Read the model definition and answer for the solid it produces. Units are mm, in the model's axes. A direction names the side the tool comes from. Coordinates: 2 decimals unless noted, no trailing zeros. Write each loop counter-clockwise with the first axis right and the second up, starting at its lowest first coordinate (ties: lowest second). Pieces come first, ordered by that corner, then holes. Notation, with made-up numbers: (-1.75, 41) -> (55.25, 41) arc R20 ccw to (55.25, 61) -> close; hole circle Ø7 at (2, 67). An arc over 180 degrees is marked (long way). One line per item, written item: value. Start each with the question number.
1. Find section B-B, the plane y = -48. Write down the section's boundary in (x, z), and give its area (3 significant figures).
2. Find section D-D, the plane y = -9. Write down the section's boundary in (x, z).
3. Given P1, Ø5, axis at x = 12.5, z = 7, coming from the +Y side; P2, Ø6.5, axis at y = -29.5, z = 1.5, coming from the +X side; P3, Ø3, axis at y = -11, z = 0, coming from the -X side, each flat-ended and moving along its own axis, determine where each tip first touches the part or whether it passes through.
4. For faces 5 (the cylindrical face through (40.59, -24.45, 4.93)), 6 (the flat face through (0.62, -46.16, 13.51)), 7 (the cylindrical face through (0.47, -24.79, 4.93)), 8 (the flat face through (0.1, -46.7, 12.5)), determine the directions among +Z, -Z, +X, -X, +Y, -Y from which every point of the face is accessible in a straight line to the end or side of a thin tool.
5. Find section A-A, the plane z = 1. State how many separate pieces and enclosed holes the cut face has, and give its area (3 significant figures).
6. Consider line 1 along Y through (x, z) = (38.5, 2.25); line 2 along Y through (x, z) = (36, 6); line 3 along Z through (x, y) = (9, -45.5). Determine where each line is inside the solid, lowest interval first.
7. Find section C-C, the plane x = 37. Write down the section's boundary in (y, z).
8. For a pull along X with two mould halves and no side action, classify faces 1 (the flat face through (21, 0, 5)), 2 (the flat face through (41, -12, 5)), 3 (the flat face through (9.5, -36.8, 0)), 4 (the cylindrical face through (41.503, -24.861, 4.93)) as pulls with the +X half, pulls with the -X half, needs draft (parallel to the pull), parting line crosses it, or undercut.
```python
from build123d import *

# Parameters (mm, degrees)
F1_DEPTH  = 10
F3_DEPTH  = 2
F4_R      = 1.1
F5_DEPTH  = 0.6
F6_R      = 1.1
F7_DEPTH  = 0.6
F13_DEPTH = 14
F14_W     = 8
F14_H     = 1.5
F15_DEPTH = 1
F16_SIZE  = 0.5
F17_W     = 8
F17_H     = 1.5
F18_DEPTH = 1
F19_SIZE  = 0.5
F21_DEPTH = 2.5
F23_DEPTH = 1.5
F25_DEPTH = 1.5


with BuildPart() as f1:
    # F0 (on Top) → F1 (new body)
    with BuildSketch(Plane.XY):
        with BuildLine():
            Line((21, 0), (2, 0))
            ThreePointArc((2, 0), (0.5857864376, -0.5857864376), (0, -2))
            Line((0, -2), (0, -22.0858455487))
            ThreePointArc((0, -22.0858455487), (0.4831818119, -24.8239916965), (1.8743610817, -27.2313822401))
            Line((1.8743610817, -27.2313822401), (14.8743610817, -42.7075727163))
            ThreePointArc((14.8743610817, -42.7075727163), (17.6209685952, -44.8133908477), (21, -45.5620360249))
            Line((21, -45.5620360249), (21, -44.5620360249))
            ThreePointArc((21, -44.5620360249), (18.0433475208, -43.9069714948), (15.6400659465, -42.0643806299))
            Line((15.6400659465, -42.0643806299), (2.6400659465, -26.5881901537))
            ThreePointArc((2.6400659465, -26.5881901537), (1.4227840854, -24.481723428), (1, -22.0858455487))
            Line((1, -22.0858455487), (1, -2))
            ThreePointArc((1, -2), (1.2928932188, -1.2928932188), (2, -1))
            Line((2, -1), (21, -1))
            Line((21, -1), (21, 0))
        make_face()
        with BuildLine():
            Line((40, 0), (21, 0))
            Line((21, 0), (21, -1))
            Line((21, -1), (40, -1))
            ThreePointArc((40, -1), (40.7071067812, -1.2928932188), (41, -2))
            Line((41, -2), (41, -22.0858455487))
            ThreePointArc((41, -22.0858455487), (40.5772159146, -24.481723428), (39.3599340535, -26.5881901537))
            Line((39.3599340535, -26.5881901537), (26.3599340535, -42.0643806299))
            ThreePointArc((26.3599340535, -42.0643806299), (23.9566524792, -43.9069714948), (21, -44.5620360249))
            Line((21, -44.5620360249), (21, -45.5620360249))
            ThreePointArc((21, -45.5620360249), (24.3790314048, -44.8133908477), (27.1256389183, -42.7075727163))
            Line((27.1256389183, -42.7075727163), (40.1256389183, -27.2313822401))
            ThreePointArc((40.1256389183, -27.2313822401), (41.5168181881, -24.8239916965), (42, -22.0858455487))
            Line((42, -22.0858455487), (42, -2))
            ThreePointArc((42, -2), (41.4142135624, -0.5857864376), (40, 0))
        make_face()
    extrude(amount=F1_DEPTH)

    # F2 (on Top) → F3 (join)
    with BuildSketch(Plane.XY):
        with BuildLine():
            Line((46, -45), (46, 4))
            Line((46, 4), (-4, 4))
            Line((-4, 4), (-4, -45))
            Line((-4, -45), (11.3115416225, -60.7183050371))
            ThreePointArc((11.3115416225, -60.7183050371), (20.5, -65), (29.6884583775, -60.7183050371))
            Line((29.6884583775, -60.7183050371), (46, -45))
        make_face()
    extrude(amount=-F3_DEPTH)

    # F4 (on face) → F5 (join, symmetric)
    with BuildSketch(Plane.YZ.offset(46)):
        with Locations((2.9, -0.9)):
            Circle(F4_R)
    extrude(amount=F5_DEPTH, both=True)

    # F6 (on face) → F7 (join, symmetric)
    with BuildSketch(Plane(origin=(-4, 0, 0), x_dir=(0, -1, 0), z_dir=(-1, 0, 0))):
        with Locations((-2.9, -0.9)):
            Circle(F6_R)
    extrude(amount=F7_DEPTH, both=True)

    # F8 (on face) → F9 (revolve)
    with BuildSketch(Plane(origin=(-4.6, 0, 0), x_dir=(0, -1, 0), z_dir=(-1, 0, 0))):
        with BuildLine():
            Line((-2.9, -2), (-2.9, 0.2))
            ThreePointArc((-2.9, 0.2), (-4, -0.9), (-2.9, -2))
        make_face()
    revolve(axis=Axis((-4.6, 2.9, -0.9), (0, 0, 1)))

    # F10 (on face) → F11 (revolve)
    with BuildSketch(Plane.YZ.offset(46.6)):
        with BuildLine():
            Line((2.9, -2), (2.9, 0.2))
            ThreePointArc((2.9, 0.2), (1.8, -0.9), (2.9, -2))
        make_face()
    revolve(axis=Axis((46.6, 2.9, -0.9), (0, 0, 1)))

    # F12 (on face) → F13 (join)
    with BuildSketch(Plane.XY):
        with BuildLine():
            Line((-2.9255281827, -43.9533337142), (-4, -45))
            Line((-4, -45), (11.3115416225, -60.7183050371))
            ThreePointArc((11.3115416225, -60.7183050371), (20.5, -65), (29.6884583775, -60.7183050371))
            Line((29.6884583775, -60.7183050371), (46, -45))
            Line((46, -45), (44.9249905697, -43.9528100137))
            Line((44.9249905697, -43.9528100137), (28.5888193042, -59.6948489351))
            ThreePointArc((28.5888193042, -59.6948489351), (20.5114901112, -63.4999937132), (12.4258523564, -59.7125360207))
            Line((12.4258523564, -59.7125360207), (-2.9255281827, -43.9533337142))
        make_face()
    extrude(amount=F13_DEPTH)

    # F14 (on face) → F15 (join)
    with BuildSketch(Plane(origin=(43.5920408851, -45.2372814773, 0), x_dir=(-0.7200798684, -0.6938911897, 0), z_dir=(-0.6938911897, 0.7200798684, 0))):
        with Locations((2.1488863345, 13.25)):
            Rectangle(F14_W, F14_H)
    extrude(amount=F15_DEPTH)

    # F16
    f16_edges = [f1.edges().sort_by_distance(p)[0] for p in [
        (41.35078, -46.008295, 12.5),
    ]]
    chamfer(f16_edges, length=F16_SIZE)

    # F17 (on face) → F18 (join)
    with BuildSketch(Plane(origin=(-23.4702228156, -22.8628527493, 0), x_dir=(-0.6977775239, 0.7163145449, 0), z_dir=(0.7163145449, 0.6977775239, 0))):
        with Locations((-33.4430444229, 13.25)):
            Rectangle(F17_W, F17_H)
    extrude(amount=F18_DEPTH)

    # F19
    f19_edges = [f1.edges().sort_by_distance(p)[0] for p in [
        (0.581896, -46.120814, 12.5),
    ]]
    chamfer(f19_edges, length=F19_SIZE)

    # F20 (on face) → F21 (join)
    with BuildSketch(Plane.XY.offset(14)):
        with BuildLine():
            ThreePointArc((29.6884583775, -60.7183050371), (20.5, -65), (11.3115416225, -60.7183050371))
            Line((11.3115416225, -60.7183050371), (9.3972794606, -62.3262852531))
            ThreePointArc((9.3972794606, -62.3262852531), (20.5, -67.5), (31.6027205394, -62.3262852531))
            Line((31.6027205394, -62.3262852531), (29.6884583775, -60.7183050371))
        make_face()
    extrude(amount=-F21_DEPTH)

    # F22 (on face) → F23 (join)
    with BuildSketch(Plane.YZ.offset(46)):
        Polygon((-45, 4), (-45, 0), (-30, 0), align=None)
    extrude(amount=-F23_DEPTH)

    # F24 (on face) → F25 (join)
    with BuildSketch(Plane(origin=(-4, 0, 0), x_dir=(0, -1, 0), z_dir=(-1, 0, 0))):
        Polygon((30, 0), (45, 0), (45, 4), align=None)
    extrude(amount=-F25_DEPTH)


solid = f1.part
```
Answer block:
1. outline: (-1.08, -2) -> (42.89, -2) -> (42.89, 14) -> (39.28, 14) -> (39.28, 13) -> (40, 12.5) -> (40.73, 12.5) -> (40.73, 0) -> (1.02, 0) -> (1.02, 12.5) -> (1.71, 12.5) -> (2.41, 13) -> (2.41, 14) -> (-1.08, 14) -> close
1. area: 151 mm2
2. outline: (-4, -2) -> (46, -2) -> (46, 0) -> (42, 0) -> (42, 10) -> (41, 10) -> (41, 0) -> (1, 0) -> (1, 10) -> (0, 10) -> (0, 0) -> (-4, 0) -> close
3. P1: stops at y = 0
3. P2: stops at x = 46
3. P3: stops at x = -4
4. face 5: +Z
4. face 6: +Z, +Y
4. face 7: +Z, -X
4. face 8: +Y
5. separate pieces: 2
5. enclosed holes: 1
5. area: 275 mm2
6. line 1: y = -52.23 to -50.14, -29.17 to -27.61, -1 to 0
6. line 2: y = -54.64 to -52.55, -32.14 to -30.59, -1 to 0
6. line 3: z = -2 to 0
7. outline: (-53.67, -2) -> (4, -2) -> (4, 0) -> (0, 0) -> (0, 10) -> (-1, 10) -> (-1, 0) -> (-29.4, 0) -> (-29.4, 10) -> (-30.95, 10) -> (-30.95, 0) -> (-51.59, 0) -> (-51.59, 14) -> (-53.67, 14) -> close
8. face 1: needs draft
8. face 2: undercut
8. face 3: undercut
8. face 4: pulls with the +X half
